Geometry check sheet. Reference: the model listing, model coordinates, mm. A direction names the side the tool comes from. Round coordinates to 2 decimals unless told otherwise and drop trailing zeros. Write each loop counter-clockwise with the first axis right and the second up, starting at its lowest first coordinate (ties: lowest second). Pieces come first, ordered by that corner, then holes. Notation, with made-up numbers: (88.5, 8.25) - (140.5, 8.25) arc R25 ccw to (140.5, 24.25) - close; hole circle Ø11 at (55.25, -36.5). An arc over 180 degrees is marked (long way). Return JSON: item names as keys, results as strings. Group by question number.
from build123d import *

# Parameters (mm, degrees)
SKETCH_1_R          = 8.5
EXTRUDE_1_DEPTH     = 12
SKETCH_2_R          = 1
CUT_EXTRUDE_1_DEPTH = 20
CUT_EXTRUDE_2_DEPTH = 8
SKETCH_4_R          = 4.4
CUT_EXTRUDE_3_DEPTH = 2
SKETCH_5_R          = 2
CUT_EXTRUDE_4_DEPTH = 4


with BuildPart() as part:
    # ｽｹｯﾁ1 → ﾎﾞｽ - 押し出し1 (new body)
    with BuildSketch(Plane.XY):
        Circle(SKETCH_1_R)
    extrude(amount=EXTRUDE_1_DEPTH)

    # ｽｹｯﾁ2 → ｶｯﾄ - 押し出し1 (cut)
    with BuildSketch(Plane.XY.offset(12)):
        with Locations((0, 6)):
            Circle(SKETCH_2_R)
        with Locations((4.242640687, 4.242640687)):
            Circle(SKETCH_2_R)
        with Locations((6, 0)):
            Circle(SKETCH_2_R)
        with Locations((4.242640687, -4.242640687)):
            Circle(SKETCH_2_R)
        with Locations((0, -6)):
            Circle(SKETCH_2_R)
        with Locations((-4.242640687, -4.242640687)):
            Circle(SKETCH_2_R)
        with Locations((-6, 0)):
            Circle(SKETCH_2_R)
        with Locations((-4.242640687, 4.242640687)):
            Circle(SKETCH_2_R)
    extrude(amount=-CUT_EXTRUDE_1_DEPTH, mode=Mode.SUBTRACT)

    # ｽｹｯﾁ3 → ｶｯﾄ - 押し出し2 (cut)
    with BuildSketch(Plane.XY.offset(12)):
        Polygon((0, 1.5), (-1.299038106, 0.75), (-1.299038106, -0.75), (0, -1.5), (1.299038106, -0.75), (1.299038106, 0.75), align=None)
    extrude(amount=-CUT_EXTRUDE_2_DEPTH, mode=Mode.SUBTRACT)

    # ｽｹｯﾁ4 → ｶｯﾄ - 押し出し3 (cut)
    with BuildSketch(Plane(origin=(0, 0, 0), x_dir=(-1, 0, 0), z_dir=(0, 0, -1))):
        Circle(SKETCH_4_R)
    extrude(amount=-CUT_EXTRUDE_3_DEPTH, mode=Mode.SUBTRACT)

    # ｽｹｯﾁ5 → ｶｯﾄ - 押し出し4 (cut)
    with BuildSketch(Plane.XY.offset(12)):
        with Locations((0, 6)):
            Circle(SKETCH_5_R)
        with Locations((4.242640687, 4.242640687)):
            Circle(SKETCH_5_R)
        with Locations((6, 0)):
            Circle(SKETCH_5_R)
        with Locations((4.242640687, -4.242640687)):
            Circle(SKETCH_5_R)
        with Locations((0, -6)):
            Circle(SKETCH_5_R)
        with Locations((-4.242640687, -4.242640687)):
            Circle(SKETCH_5_R)
        with Locations((-6, 0)):
            Circle(SKETCH_5_R)
        with Locations((-4.242640687, 4.242640687)):
            Circle(SKETCH_5_R)
    extrude(amount=-CUT_EXTRUDE_4_DEPTH, mode=Mode.SUBTRACT)


solid = part.part
1. Section check A-A (y = 0). Enter the section's corners in (x, z), and give its area (3 significant figures).
2. Depth check by flat-ended pin: pin 1 Ø1 at (x, y) = (-4.5, 7) entering from -Z; pin 2 Ø5 at (x, z) = (5.5, 1.5) entering from -Y; pin 3 Ø2 at (y, z) = (-3.5, 3.5) entering from -X; pin 4 Ø4 at (y, z) = (2.5, 10) entering from +X. Enter the tip coordinate at first touch or a pass-through.
3. Section check D-D (x = 0.5). Enter the section's corners in (y, z).
4. Section check C-C (y = -6). Enter the section's corners in (x, z), and give its area (3 significant figures).
5. Section check B-B (z = 7.75). State how many separate pieces and enclosed holes the cut face has, and give its area (3 significant figures).
6. Material ranges on line 1 along Y through (x, z) = (0, 2.75); line 2 along X through (y, z) = (3.75, 1); line 3 along X through (y, z) = (3.5, 3.5), recorded low to high.
7. Tool access check on faces 1 (the face through (-1.299, 0, 8)), 2 (the face through (-3.32, -4.63, 4.06)), 3 (the face through (-4.197, 1.322, 0.986)). Record the directions out of +Z, -Z, +X, -X, +Y, -Y that give a thin tool (end or side, any length) a straight path to the whole face; none if there is none.
Result sheet:
{
 "1": {"outline": "(-8.5, 0) - (-7, 0) - (-7, 8) - (-8, 8) - (-8, 12) - (-8.5, 12) - close; (-5, 0) - (-4.4, 0) - (-4.4, 2) - (4.4, 2) - (4.4, 0) - (5, 0) - (5, 8) - (4, 8) - (4, 12) - (1.3, 12) - (1.3, 4) - (-1.3, 4) - (-1.3, 12) - (-4, 12) - (-4, 8) - (-5, 8) - close; (7, 0) - (8.5, 0) - (8.5, 12) - (8, 12) - (8, 8) - (7, 8) - close", "area": "102 mm²"},
 "2": {"pin 1": "stops at z = 0", "pin 2": "stops at y = -7.95", "pin 3": "stops at x = -8.12", "pin 4": "stops at x = 8.49"},
 "3": {"outline": "(-8.49, 0) - (-6.87, 0) - (-6.87, 8) - (-7.94, 8) - (-7.94, 12) - (-8.49, 12) - close; (-5.13, 0) - (-4.37, 0) - (-4.37, 2) - (4.37, 2) - (4.37, 0) - (5.13, 0) - (5.13, 8) - (4.06, 8) - (4.06, 12) - (1.21, 12) - (1.21, 4) - (-1.21, 4) - (-1.21, 12) - (-4.06, 12) - (-4.06, 8) - (-5.13, 8) - close; (6.87, 0) - (8.49, 0) - (8.49, 12) - (7.94, 12) - (7.94, 8) - (6.87, 8) - close"},
 "4": {"outline": "(-6.02, 0) - (-1, 0) - (-1, 8) - (-2, 8) - (-2, 12) - (-3.29, 12) - (-3.29, 8) - (-5.2, 8) - (-5.2, 12) - (-6.02, 12) - close; (1, 0) - (6.02, 0) - (6.02, 12) - (5.2, 12) - (5.2, 8) - (3.29, 8) - (3.29, 12) - (2, 12) - (2, 8) - (1, 8) - close", "area": "97.2 mm²"},
 "5": {"separate pieces": "1", "enclosed holes": "9", "area": "196 mm²"},
 "6": {"line 1": "y = -8.5 to -7, -5 to 5, 7 to 8.5", "line 2": "x = -7.63 to -5.11, -3.37 to -2.3, 2.3 to 3.37, 5.11 to 7.63", "line 3": "x = -7.75 to -4.91, -3.57 to 3.57, 4.91 to 7.75"},
 "7": {"face 1": "+Z", "face 2": "+Z, -Z", "face 3": "-Z"}
}
